from build123d import *

# Parameters (mm, degrees)
SKETCH_1_W               = 80.2
SKETCH_1_H               = 40.6
SKETCH_1_R               = 9.4
SKETCH_1_R_2             = 2.5
EXTRUDE_1_DEPTH          = 6
SKETCH_2_W               = 80.2
SKETCH_2_H               = 40.6
EXTRUDE_2_DEPTH          = 3
SKETCH_3_W               = 80.2
SKETCH_3_H               = 8.4
CUT_EXTRUDE_1_DEPTH      = 3
SKETCH_4_W               = 8.8
SKETCH_4_H               = 40.6
CUT_EXTRUDE_2_DEPTH      = 3
SKETCH_5_R               = 2.5
SKETCH_5_R_2             = 1.5
CUT_EXTRUDE_3_DEPTH      = 7
CUT_EXTRUDE_3_DEPTH_BACK = 10
FILLET_3_R               = 5
FILLET_8_R               = 5
FILLET_9_R               = 5
FILLET_10_R              = 5


with BuildPart() as part:
    # 草图1 → 凸台-拉伸1 (new body)
    with BuildSketch(Plane.XY):
        with Locations((29.7, -9.9)):
            Rectangle(SKETCH_1_W, SKETCH_1_H)
        Circle(SKETCH_1_R, mode=Mode.SUBTRACT)
        with Locations((19.8, 0)):
            Circle(SKETCH_1_R, mode=Mode.SUBTRACT)
        with Locations((39.6, 0)):
            Circle(SKETCH_1_R, mode=Mode.SUBTRACT)
        with Locations((59.4, 0)):
            Circle(SKETCH_1_R, mode=Mode.SUBTRACT)
        with Locations((0, -19.8)):
            Circle(SKETCH_1_R, mode=Mode.SUBTRACT)
        with Locations((19.8, -19.8)):
            Circle(SKETCH_1_R, mode=Mode.SUBTRACT)
        with Locations((39.6, -19.8)):
            Circle(SKETCH_1_R, mode=Mode.SUBTRACT)
        with Locations((59.4, -19.8)):
            Circle(SKETCH_1_R, mode=Mode.SUBTRACT)
        with Locations((9.9, -9.9)):
            Circle(SKETCH_1_R_2, mode=Mode.SUBTRACT)
        with Locations((29.7, -9.9)):
            Circle(SKETCH_1_R_2, mode=Mode.SUBTRACT)
        with Locations((49.5, -9.9)):
            Circle(SKETCH_1_R_2, mode=Mode.SUBTRACT)
    extrude(amount=EXTRUDE_1_DEPTH)

    # 草图2 → 凸台-拉伸2 (add)
    with BuildSketch(Plane.XY.offset(6)):
        with Locations((29.7, -9.9)):
            Rectangle(SKETCH_2_W, SKETCH_2_H)
    extrude(amount=EXTRUDE_2_DEPTH)

    # 草图3 → 切除-拉伸1 (cut)
    with BuildSketch(Plane.XY.offset(9)):
        with Locations((29.7, -0.18)):
            Rectangle(SKETCH_3_W, SKETCH_3_H)
        with Locations((29.7, -19.62)):
            Rectangle(SKETCH_3_W, SKETCH_3_H)
    extrude(amount=-CUT_EXTRUDE_1_DEPTH, mode=Mode.SUBTRACT)

    # 草图4 → 切除-拉伸2 (cut)
    with BuildSketch(Plane.XY.offset(9)):
        with Locations((0, -9.9)):
            Rectangle(SKETCH_4_W, SKETCH_4_H)
        with Locations((19.8, -9.9)):
            Rectangle(SKETCH_4_W, SKETCH_4_H)
        with Locations((39.6, -9.9)):
            Rectangle(SKETCH_4_W, SKETCH_4_H)
        with Locations((59.4, -9.9)):
            Rectangle(SKETCH_4_W, SKETCH_4_H)
    extrude(amount=-CUT_EXTRUDE_2_DEPTH, mode=Mode.SUBTRACT)

    # 草图5 → 切除-拉伸3 (cut, two sides)
    with BuildSketch(Plane(origin=(0, 0, 6), x_dir=(-1, 0, 0), z_dir=(0, 0, -1))) as cut_extrude_3_sk:
        with Locations((-49.5, -9.9)):
            Circle(SKETCH_5_R)
        with Locations((-29.7, -9.9)):
            Circle(SKETCH_5_R)
        with Locations((-9.9, -9.9)):
            Circle(SKETCH_5_R)
        with Locations((-66.76305517, -9.9)):
            Circle(SKETCH_5_R_2)
        with Locations((7.36305517, -9.9)):
            Circle(SKETCH_5_R_2)
    extrude(amount=CUT_EXTRUDE_3_DEPTH, mode=Mode.SUBTRACT)
    extrude(cut_extrude_3_sk.sketch, amount=-CUT_EXTRUDE_3_DEPTH_BACK, mode=Mode.SUBTRACT)

    # 圆角3
    fillet_3_edges = [part.edges().sort_by_distance(p)[0] for p in [
        (-10.4, -30.2, 4.5),
    ]]
    fillet(fillet_3_edges, radius=FILLET_3_R)

    # 圆角8
    fillet_8_edges = [part.edges().sort_by_distance(p)[0] for p in [
        (69.8, -30.2, 4.5),
    ]]
    fillet(fillet_8_edges, radius=FILLET_8_R)

    # 圆角9
    fillet_9_edges = [part.edges().sort_by_distance(p)[0] for p in [
        (69.8, 10.4, 4.5),
    ]]
    fillet(fillet_9_edges, radius=FILLET_9_R)

    # 圆角10
    fillet_10_edges = [part.edges().sort_by_distance(p)[0] for p in [
        (-10.4, 10.4, 4.5),
    ]]
    fillet(fillet_10_edges, radius=FILLET_10_R)


solid = part.part
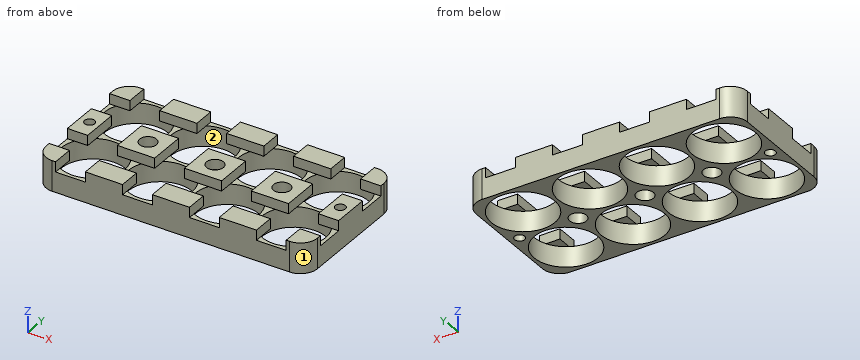
Can you work these out from the model? Positions are in its coordinate system, mm. Face numbers are marked on the shaded views. A direction names the side the tool comes from. Give positions to 0.01 mm unless a question says otherwise; leave off trailing zeros. Loops run counter-clockwise (first coordinate to the right, second up) from the corner with the lowest first, then second, coordinate; pieces in that order, holes last. Notation, with made-up numbers: (77.25, 19) -> (81.25, 19) arc R26 ccw to (81.25, 41) -> close; hole circle Ø10 at (45, -5). An arc over 180 degrees is marked (long way). Use one line per item in the form item = value.
1) If we section it at C-C (x = 59.4): Please give me the cut outline in (y, z), plus the area to 3 significant figures.
Answers:
outline = (-30.2, 0) -> (-29.2, 0) -> (-29.2, 6) -> (-30.2, 6) -> close; (-10.4, 0) -> (-9.4, 0) -> (-9.4, 6) -> (-10.4, 6) -> close; (9.4, 0) -> (10.4, 0) -> (10.4, 6) -> (9.4, 6) -> close
area = 18.0 mm²
2) For the marked faces 1 and 2, which set-ups out of +Z, -Z, +X, -X, +Y, -Y let a thin tool reach every point of the face, with its end or its side?
Answers:
face_1 = +Z, -Z, +X, -Y
face_2 = -Z
3) I need wall thicknesses on line 1 along Y through (x, z) = (49.5, 8); line 2 along X through (y, z) = (0, 4.75); line 3 along X through (y, z) = (-9.9, 3.1). Which ranges of each line are inside material? Lowest first, please.
Answers:
line_1 = -30.2 to -23.82, -15.42 to -12.4, -7.4 to -4.38, 4.02 to 10.4
line_2 = -10.4 to -9.4, 9.4 to 10.4, 29.2 to 30.2, 49 to 50, 68.8 to 69.8
line_3 = -10.4 to -8.86, -5.86 to 7.4, 12.4 to 27.2, 32.2 to 47, 52 to 65.26, 68.26 to 69.8
4) If we section it at B-B (z = 3.25): Count the separate pieces of the cut face and the enclosed holes in it, plus the area to 3 significant figures.
Answers:
separate_pieces = 1
enclosed_holes = 13
area = 941 mm²
5) Will these pins go through, and if not, where does the flat tip stop? pin 1 (2.5 mm diameter, centred on y = -27.5, z = 8, fed in from +X); pin 2 (3.5 mm diameter, centred on x = 20, y = -10.5, fed in from +Z); pin 3 (11.5 mm diameter, centred on x = 39.6, y = 0, fed in from +Z); pin 4 (1.5 mm diameter, centred on y = 7, z = 8, fed in from -X).
Answers:
pin_1 = 69.69
pin_2 = 6
pin_3 = through
pin_4 = -10.33
6) If we section it at A-A (y = -19.8): Please give me the cut outline in (x, z).
Answers:
outline = (-10.4, 0) -> (-9.4, 0) -> (-9.4, 6) -> (-10.4, 6) -> close; (9.4, 0) -> (10.4, 0) -> (10.4, 6) -> (9.4, 6) -> close; (29.2, 0) -> (30.2, 0) -> (30.2, 6) -> (29.2, 6) -> close; (49, 0) -> (50, 0) -> (50, 6) -> (49, 6) -> close; (68.8, 0) -> (69.8, 0) -> (69.8, 6) -> (68.8, 6) -> close
